from build123d import *

# Parameters (mm, degrees)
BOSS_EXTRUDE1_DEPTH = 11.7856
FILLET1_R           = 2.54
CHAMFER1_SIZE       = 2.54


with BuildPart() as part:
    # Sketch1 → Boss-Extrude1 (new body)
    with BuildSketch(Plane(origin=(0, 0, 0), x_dir=(1, 0, 0), z_dir=(0, 1, 0))):
        Polygon((-55.35295, 32.6136), (55.35295, 32.6136), (55.35295, -32.6136), (-55.35295, -32.6136), (-55.35295, -6.17855), (-62.13475, -6.17855), (-62.13475, 0), (-62.13475, 6.17855), (-55.35295, 6.17855), align=None)
    extrude(amount=BOSS_EXTRUDE1_DEPTH)

    # Fillet1
    fillet1_edges = [part.edges().sort_by_distance(p)[0] for p in [
        (-55.35295, 0, -19.396075),
        (0, 0, -32.6136),
        (55.35295, 0, 0),
        (55.35295, 5.8928, 32.6136),
        (-55.35295, 5.8928, 32.6136),
        (-55.35295, 5.8928, -32.6136),
        (55.35295, 5.8928, -32.6136),
        (0, 0, 32.6136),
        (-55.35295, 0, 19.396075),
    ]]
    fillet(fillet1_edges, radius=FILLET1_R)

    # Chamfer1
    chamfer1_edges = [part.edges().sort_by_distance(p)[0] for p in [
        (-62.13475, 5.8928, 6.17855),
        (-62.13475, 5.8928, -6.17855),
    ]]
    chamfer(chamfer1_edges, length=CHAMFER1_SIZE)


solid = part.part
CAD build for the part. Positions are in the model's coordinates, mm. A direction names the side the tool comes from. Round coordinates to 2 decimals unless told otherwise and drop trailing zeros. Write each loop counter-clockwise with the first axis right and the second up, starting at its lowest first coordinate (ties: lowest second). Pieces come first, ordered by that corner, then holes.
(1) Slice it at B-B, the plane z = -21.5. Write the cut outline in (x, y), and give its area (3 significant figures).
(2) Probe line 1 along Z through (x, y) = (-56, 10.5); line 2 along X through (y, z) = (6.5, 10.5); line 3 along X through (y, z) = (0.5, 22). List the from-to ranges inside material, lowest first.
(3) 3-axis set-ups, long thin cutter, end or side, ignore diameter. For faces 1 (the face through (-55.353, 7, -18)), 2 (the face through (-54.629, 0.764, -18.293)), 3 (the face through (-54.629, 0.764, 17.959)): which of +Z, -Z, +X, -X, +Y, -Y reach the whole face in a straight line?
(4) Drop flat-ended pins along their axis: P1, Ø6, axis at y = 3.5, z = -9.5, coming from the -X side; P2, Ø1, axis at x = 27.5, y = 1.5, coming from the -Z side. Give the stop position or say it passes through.
(5) Slice it at A-A, the plane y = 6. Write the cut outline in (x, z), and give its area (3 significant figures).
From the geometry:
1. outline: (-55.35, 2.54) arc R2.54 ccw to (-52.81, 0) - (52.81, 0) arc R2.54 ccw to (55.35, 2.54) - (55.35, 11.79) - (-55.35, 11.79) - close
1. area: 1,300 mm2
2. line 1: z = -6.18 to 6.18
2. line 2: x = -55.35 to 55.35
2. line 3: x = -54.33 to 54.33
3. face 1: -Z, -X, +Y, -Y
3. face 2: -Z, -X, -Y
3. face 3: +Z, -X, -Y
4. P1: stops at x = -55.35
4. P2: stops at z = -32.56
5. outline: (-62.13, -3.64) - (-59.59, -6.18) - (-55.35, -6.18) - (-55.35, -30.07) arc R2.54 ccw to (-52.81, -32.61) - (52.81, -32.61) arc R2.54 ccw to (55.35, -30.07) - (55.35, 30.07) arc R2.54 ccw to (52.81, 32.61) - (-52.81, 32.61) arc R2.54 ccw to (-55.35, 30.07) - (-55.35, 6.18) - (-59.59, 6.18) - (-62.13, 3.64) - close
5. area: 7,290 mm2
